from build123d import *

# Parameters (mm, degrees)
SKETCH_3_R          = 13.661879352
EXTRUDE_1_DEPTH     = 12.5
CUT_EXTRUDE_1_DEPTH = 5
FILLET_1_R          = 5


with BuildPart() as part:
    # 草图2 → 旋转1 (revolve)
    with BuildSketch(Plane.XY):
        Polygon((0, 0), (-25, 0), (-25, 20), (-10, 20), (-10, 60), (-25, 60), (-25, 80), (0, 80), align=None)
    revolve(axis=Axis((0, 80, 0), (0, -1, 0)))

    # 草图3 → 凸台-拉伸1 (add, symmetric)
    with BuildSketch(Plane(origin=(0, 40, 0), x_dir=(1, 0, 0), z_dir=(0, 1, 0))):
        with Locations(Location((0, 0, 0), (0, 0, 180))):
            Circle(SKETCH_3_R)
    extrude(amount=EXTRUDE_1_DEPTH, both=True)

    # 草图4 → 切除-拉伸1 (cut)
    with BuildSketch(Plane(origin=(0, 80, 0), x_dir=(1, 0, 0), z_dir=(0, 1, 0))):
        with BuildLine():
            Line((-3.834152171, -8.865208988), (-3.834152171, 8.865208988))
            ThreePointArc((-3.834152171, 8.865208988), (0, 12.699361159), (3.834152171, 8.865208988))
            Line((3.834152171, 8.865208988), (3.834152171, -8.865208988))
            ThreePointArc((3.834152171, -8.865208988), (0, -12.699361159), (-3.834152171, -8.865208988))
        make_face()
    extrude(amount=-CUT_EXTRUDE_1_DEPTH, mode=Mode.SUBTRACT)

    # 草图5 → 切除-旋转1 (revolve, cut)
    with BuildSketch(Plane(origin=(0, 0, 0), x_dir=(0, 0, -1), z_dir=(1, 0, 0)), mode=Mode.PRIVATE) as cut_revolve_1_sk:
        Polygon((-25, 80), (-25, 76.608006346), (-21.608006346, 80), align=None)
    revolve(cut_revolve_1_sk.sketch.rotate(Axis((0, 0, 0), (0, 1, 0)), 270), axis=Axis((0, 0, 0), (0, 1, 0)), mode=Mode.SUBTRACT)

    # 圆角1
    # the kernel refuses this fillet: 5 mm, written as the material it takes off along each edge
    with BuildSketch(Plane(origin=(0, 27.5, 0), x_dir=(-1, 0, 0), z_dir=(0, 0, -1))) as fillet_1_piece_1:
        with BuildLine():
            CenterArc((8.661879352, 4.817616956), FILLET_1_R, 285.5229375, 74.4770625)
            Line((13.661879352, 4.817616956), (13.761879352, 4.817616956))
            Line((13.761879352, 4.817616956), (13.761879352, 0))
            Line((13.761879352, 0), (13.661879352, -0.1))
            ThreePointArc((13.661879352, -0.1), (11.830939676, -0.1), (10.026762413, -0.096352339))
            Line((10.026762413, -0.096352339), (10, 0))
        make_face()
    revolve(axis=Axis((0, 27.5, 0), (0, 1, 0)), mode=Mode.SUBTRACT)
    with BuildSketch(Plane(origin=(0, 52.5, 0), x_dir=(-1, 0, 0), z_dir=(0, 0, -1))) as fillet_1_piece_2:
        with BuildLine():
            CenterArc((8.661879352, -4.817616956), FILLET_1_R, 0, 74.4770625)
            Line((10, 0), (10.026762413, 0.096352339))
            ThreePointArc((10.026762413, 0.096352339), (11.830939676, 0.1), (13.661879352, 0.1))
            Line((13.661879352, 0.1), (13.761879352, 0))
            Line((13.761879352, 0), (13.761879352, -4.817616956))
            Line((13.761879352, -4.817616956), (13.661879352, -4.817616956))
        make_face()
    revolve(axis=Axis((0, 52.5, 0), (0, 1, 0)), mode=Mode.SUBTRACT)
    with BuildSketch(Plane(origin=(0, 60, 0), x_dir=(-1, 0, 0), z_dir=(0, 0, 1))) as fillet_1_piece_3:
        with BuildLine():
            CenterArc((25 - FILLET_1_R, -FILLET_1_R), FILLET_1_R, 0, 90)
            Line((25, -FILLET_1_R), (25 + FILLET_1_R * 0.02, -FILLET_1_R))
            Line((25 + FILLET_1_R * 0.02, -FILLET_1_R), (25 + FILLET_1_R * 0.02, FILLET_1_R * 0.02))
            Line((25 + FILLET_1_R * 0.02, FILLET_1_R * 0.02), (25 - FILLET_1_R, FILLET_1_R * 0.02))
            Line((25 - FILLET_1_R, FILLET_1_R * 0.02), (25 - FILLET_1_R, 0))
        make_face()
    revolve(axis=Axis((0, 60, 0), (0, -1, 0)), mode=Mode.SUBTRACT)
    with BuildSketch(Plane(origin=(0, 20, 0), x_dir=(-1, 0, 0), z_dir=(0, 0, 1))) as fillet_1_piece_4:
        with BuildLine():
            CenterArc((25 - FILLET_1_R, FILLET_1_R), FILLET_1_R, 270, 90)
            Line((25 - FILLET_1_R, 0), (25 - FILLET_1_R, -FILLET_1_R * 0.02))
            Line((25 - FILLET_1_R, -FILLET_1_R * 0.02), (25 + FILLET_1_R * 0.02, -FILLET_1_R * 0.02))
            Line((25 + FILLET_1_R * 0.02, -FILLET_1_R * 0.02), (25 + FILLET_1_R * 0.02, FILLET_1_R))
            Line((25 + FILLET_1_R * 0.02, FILLET_1_R), (25, FILLET_1_R))
        make_face()
    revolve(axis=Axis((0, 20, 0), (0, -1, 0)), mode=Mode.SUBTRACT)
    with BuildSketch(Plane(origin=(0, 0, 0), x_dir=(-1, 0, 0), z_dir=(0, 0, 1))) as fillet_1_piece_5:
        with BuildLine():
            CenterArc((25 - FILLET_1_R, -FILLET_1_R), FILLET_1_R, 0, 90)
            Line((25, -FILLET_1_R), (25 + FILLET_1_R * 0.02, -FILLET_1_R))
            Line((25 + FILLET_1_R * 0.02, -FILLET_1_R), (25 + FILLET_1_R * 0.02, FILLET_1_R * 0.02))
            Line((25 + FILLET_1_R * 0.02, FILLET_1_R * 0.02), (25 - FILLET_1_R, FILLET_1_R * 0.02))
            Line((25 - FILLET_1_R, FILLET_1_R * 0.02), (25 - FILLET_1_R, 0))
        make_face()
    revolve(axis=Axis((0, 0, 0), (0, -1, 0)), mode=Mode.SUBTRACT)


solid = part.part
Part model, mm, in its own coordinate system. A direction names the side the tool comes from. Coordinates: 2 decimals unless noted, no trailing zeros. Order: outer loops, then holes, each group sorted by start corner. A loop starts at its lowest first (then second) coordinate and runs counter-clockwise, first axis right, second up. Notation, with made-up numbers: M -12.5,-3 L 1.5,-3 A24 cw 1.5,20 Z; hole C 71,-28 d11. An arc over 180 degrees is marked long. Use a Markdown table: item, result.
(1) Pull direction X, two halves, no side cores. Call faces 1 (the flat face through (0, 0, 0)), 2 (the cylindrical face through (-0.1, 77.5, -12.7)), 3 (the cylindrical face through (2.17, 23.8, 9.76)): released by +X, released by -X, zero draft, split by the parting line, or undercut.
A:
| item | result |
|---|---|
| face 1 | zero draft |
| face 2 | undercut |
| face 3 | split by the parting line |
(2) Cut at C-C on y = 71. Write the cut outline in (x, z).
A:
| item | result |
|---|---|
| outline | C 0,0 d50 |
(3) Tool access for faces 4 (the flat face through (5, 20, -9)), 5 (the cylindrical face through (-23.846, 70.885, -7.509)), 6 (the flat face through (-3.834, 78, 0)): list every direction of +Z, -Z, +X, -X, +Y, -Y with a clear straight run to the whole face (end or side of a thin tool).
A:
| item | result |
|---|---|
| face 4 | none |
| face 5 | +Y, -Y |
| face 6 | +Y |
(4) Flat gauge pins, fed straight in: pin 1 (3 mm diameter, centred on y = 8, z = -2.5, fed in from -X); pin 2 (6 mm diameter, centred on y = 27.5, z = 9.5, fed in from +X); pin 3 (1.5 mm diameter, centred on y = 77, z = -2.5, fed in from -X). Where does each tip first touch, or does it go through?
A:
| item | result |
|---|---|
| pin 1 | stops at x = -24.98 |
| pin 2 | stops at x = 10.55 |
| pin 3 | stops at x = -24.93 |
(5) Cut at D-D on y = 40. Write the cut outline in (x, z), then the cut area to 3 significant figures.
A:
| item | result |
|---|---|
| outline | C 0,0 d27.32 |
| area | 586 mm^2 |
(6) Probe L1, parallel to Y at x = -4.5, z = -9; L2, parallel to Y at x = -9, z = -13; L3, parallel to Y at x = -2, z = -11.5. List the from-to ranges inside material, lowest first.
A:
| item | result |
|---|---|
| L1 | y = 0 to 20, 27.52 to 52.48, 60 to 80 |
| L2 | y = 0 to 20, 60 to 80 |
| L3 | y = 0 to 20, 28.33 to 51.67, 60 to 75 |
